Source: CAD feature listing. Evaluate the final solid. Frame: model axes, mm. Face numbers are marked on the shaded views. A direction names the side the tool comes from. Coordinates: 2 decimals unless noted, no trailing zeros. Order: outer loops, then holes, each group sorted by start corner. A loop starts at its lowest first (then second) coordinate and runs counter-clockwise, first axis right, second up. Notation, with made-up numbers: (65, 7) - (122, 7) arc R26 cw to (122, 39) - close; hole circle Ø4 at (-24, 41.25). An arc over 180 degrees is marked (long way). One line per question, with ' | ' between items. Start each with the question number.
(1) Section D-D (y = 4.5). Count the separate pieces of the cut face and the enclosed holes in it, then the cut area to 3 significant figures.
(2) Access query for the marked faces 4 and 5. Directions: +Z, -Z, +X, -X, +Y, -Y. A direction counts if a zero-diameter tool reaches every point of the face in a straight line with its end or side. Return the directions, or none.
(3) Contact query for flat-ended pins moving along their axis: P1, Ø2, axis at x = 2.05, z = -1.49, coming from the -Y side (3 decimals); P2, Ø3, axis at x = 5, y = 1.5, coming from the -Z side. Output: stop coordinate, or through.
(4) Section C-C (z = -8). Return the cut outline in (x, y) (3 decimals), then the cut area to 3 significant figures.
(5) Section A-A (z = 0). Return the cut outline in (x, y) (3 decimals).
(6) Section B-B (x = 7.62). Return the cut outline in (y, z) (3 decimals), then the cut area to 3 significant figures.
(7) Draft query along X for the marked faces 1, 2 and 3. Return one class per face: +X half, -X half, draft (parallel to the pull), parting line (faces both ways), or undercut.
(8) Line query: line 1 along X through (y, z) = (4.7, 0); line 2 along X through (y, z) = (0.75, -0.25); line 3 along X through (y, z) = (5, -2). Output: solid intervals per line, ascending.
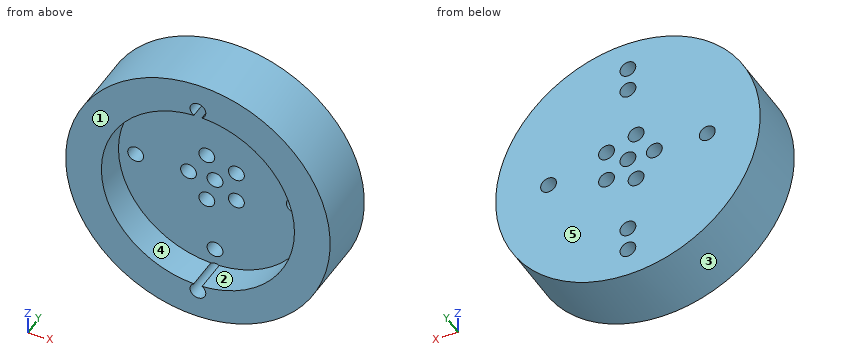
from build123d import *

# Parameters (mm, degrees)
SKETCH1_R           = 12.7
BOSS_EXTRUDE1_DEPTH = 6.35
SKETCH2_R           = 9.271
CUT_EXTRUDE1_DEPTH  = 3.175
CIRPATTERN1_COUNT   = 2
SKETCH6_R           = 0.762
CUT_EXTRUDE2_DEPTH  = 3.175


with BuildPart() as part:
    # Sketch1 → Boss-Extrude1 (new body)
    with BuildSketch(Plane(origin=(0, 0, 0), x_dir=(1, 0, 0), z_dir=(0, 1, 0))):
        with Locations(Location((0, 0, 0), (0, 0, 270))):
            Circle(SKETCH1_R)
    extrude(amount=BOSS_EXTRUDE1_DEPTH)

    # Sketch2 → Cut-Extrude1 (cut)
    with BuildSketch(Plane.XZ):
        with Locations(Location((0, 0, 0), (0, 0, 270))):
            Circle(SKETCH2_R)
    extrude(amount=-CUT_EXTRUDE1_DEPTH, mode=Mode.SUBTRACT)

    # Sketch5 → #1-72 Tapped Hole1 (revolve, cut)
    with BuildSketch(Plane(origin=(0, 0, -9.906), x_dir=(0, 0, -1), z_dir=(1, 0, 0))):
        Polygon((0, 0), (0, 11.630040327), (0.75565, 11.176), (0.75565, 0), align=None)
    f_1_72_tapped_hole1 = revolve(axis=Axis((0, -6.35, -9.906), (0, 1, 0)), mode=Mode.SUBTRACT)

    # CirPattern1: #1-72 Tapped Hole1 ×2 about axis
    cirpattern1_axis = Axis((0, 0, 0.002208913), (0, 1, 0))
    for i in range(1, CIRPATTERN1_COUNT):
        add(f_1_72_tapped_hole1.rotate(cirpattern1_axis, i * 360 / CIRPATTERN1_COUNT), mode=Mode.SUBTRACT)

    # Sketch6 → Cut-Extrude2 (cut)
    with BuildSketch(Plane(origin=(0, 6.35, 0), x_dir=(1, 0, 0), z_dir=(0, 1, 0))):
        with Locations(Location((0, 0, 0), (0, 0, 270))):
            Circle(SKETCH6_R)
        with Locations(Location((-2.54, 0, 0), (0, 0, 270))):
            Circle(SKETCH6_R)
        with Locations(Location((-0.784903166, 2.415683551, 0), (0, 0, 270))):
            Circle(SKETCH6_R)
        with Locations(Location((2.054903166, 1.492974541, 0), (0, 0, 270))):
            Circle(SKETCH6_R)
        with Locations(Location((2.054903166, -1.492974541, 0), (0, 0, 270))):
            Circle(SKETCH6_R)
        with Locations(Location((-0.784903166, -2.415683551, 0), (0, 0, 270))):
            Circle(SKETCH6_R)
        with Locations(Location((0, 7.62, 0), (0, 0, 270))):
            Circle(SKETCH6_R)
        with Locations(Location((7.62, 0, 0), (0, 0, 270))):
            Circle(SKETCH6_R)
        with Locations(Location((0, -7.62, 0), (0, 0, 270))):
            Circle(SKETCH6_R)
        with Locations(Location((-7.62, 0, 0), (0, 0, 270))):
            Circle(SKETCH6_R)
    extrude(amount=-CUT_EXTRUDE2_DEPTH, mode=Mode.SUBTRACT)


solid = part.part
Response values:
1) separate pieces: 1 | enclosed holes: 12 | area: 485 mm²
2) face 4: -Y | face 5: +Z, -Z, +X, -X, +Y
3) P1: stops at y = 3.175 | P2: stops at z = -12.21
4) outline: (-9.864, 0) - (-4.685, 0) - (-4.685, 3.175) - (-0.66, 3.175) - (-0.66, 6.35) - (-9.864, 6.35) - close; (0.66, 3.175) - (4.685, 3.175) - (4.685, 0) - (9.864, 0) - (9.864, 6.35) - (0.66, 6.35) - close | area: 91.3 mm²
5) outline: (-12.7, 0) - (-9.271, 0) - (-9.271, 3.175) - (-8.382, 3.175) - (-8.382, 6.35) - (-12.7, 6.35) - close; (-6.858, 3.175) - (-3.302, 3.175) - (-3.302, 6.35) - (-6.858, 6.35) - close; (-1.778, 3.175) - (-0.762, 3.175) - (-0.762, 6.35) - (-1.778, 6.35) - close; (0.762, 3.175) - (6.858, 3.175) - (6.858, 6.35) - (0.762, 6.35) - close; (8.382, 3.175) - (9.271, 3.175) - (9.271, 0) - (12.7, 0) - (12.7, 6.35) - (8.382, 6.35) - close
6) outline: (0, -10.16) - (6.35, -10.16) - (6.35, -0.762) - (3.175, -0.762) - (3.175, -5.281) - (0, -5.281) - close; (0, 5.281) - (3.175, 5.281) - (3.175, 0.762) - (6.35, 0.762) - (6.35, 10.16) - (0, 10.16) - close | area: 90.7 mm²
7) face 1: draft | face 2: undercut | face 3: parting line
8) line 1: x = -12.7 to -8.38, -6.86 to -3.3, -1.78 to -0.76, 0.76 to 6.86, 8.38 to 12.7 | line 2: x = -12.7 to -9.27, 9.27 to 12.7 | line 3: x = -12.54 to -1.42, -0.15 to 1.49, 2.62 to 12.54
